from build123d import *

# Parameters (mm, degrees)
SKETCH1_R           = 25
BOSS_EXTRUDE1_DEPTH = 4
SKETCH2_R           = 1.713577746
CUT_EXTRUDE1_DEPTH  = 4
CUT_EXTRUDE2_DEPTH  = 2
SKETCH4_R           = 12.5
SKETCH4_R_2         = 3
BOSS_EXTRUDE2_DEPTH = 10
SKETCH5_R           = 1.6
CUT_EXTRUDE3_DEPTH  = 12.5
SKETCH6_R           = 3.1
CUT_EXTRUDE4_DEPTH  = 6
CUT_EXTRUDE5_DEPTH  = 3
FILLET1_R           = 1.5


with BuildPart() as part:
    # Sketch1 → Boss-Extrude1 (new body)
    with BuildSketch(Plane.XY):
        Circle(SKETCH1_R)
    extrude(amount=BOSS_EXTRUDE1_DEPTH)

    # Sketch2 → Cut-Extrude1 (cut)
    with BuildSketch(Plane(origin=(0, 0, 0), x_dir=(-1, 0, 0), z_dir=(0, 0, -1))):
        with Locations((0, 18.35)):
            Circle(SKETCH2_R)
        with Locations((15.891566159, 9.175)):
            Circle(SKETCH2_R)
        with Locations((15.891566159, -9.175)):
            Circle(SKETCH2_R)
        with Locations((0, -18.35)):
            Circle(SKETCH2_R)
        with Locations((-15.891566159, -9.175)):
            Circle(SKETCH2_R)
        with Locations((-15.891566159, 9.175)):
            Circle(SKETCH2_R)
    extrude(amount=-CUT_EXTRUDE1_DEPTH, mode=Mode.SUBTRACT)

    # Sketch3 → Cut-Extrude2 (cut)
    with BuildSketch(Plane(origin=(0, 0, 0), x_dir=(-1, 0, 0), z_dir=(0, 0, -1))):
        Polygon((13.870840217, 5.675), (17.912292102, 5.675), (19.933018044, 9.175), (17.912292102, 12.675), (13.870840217, 12.675), (11.850114275, 9.175), align=None)
        Polygon((4.041451884, 18.35), (2.020725942, 21.85), (-2.020725942, 21.85), (-4.041451884, 18.35), (-2.020725942, 14.85), (2.020725942, 14.85), align=None)
        Polygon((11.850114275, -9.175), (13.870840217, -12.675), (17.912292102, -12.675), (19.933018044, -9.175), (17.912292102, -5.675), (13.870840217, -5.675), align=None)
        Polygon((-2.020725942, -14.85), (-4.041451884, -18.35), (-2.020725942, -21.85), (2.020725942, -21.85), (4.041451884, -18.35), (2.020725942, -14.85), align=None)
        Polygon((-13.870840217, -5.675), (-17.912292102, -5.675), (-19.933018044, -9.175), (-17.912292102, -12.675), (-13.870840217, -12.675), (-11.850114275, -9.175), align=None)
        Polygon((-11.850114275, 9.175), (-13.870840217, 12.675), (-17.912292102, 12.675), (-19.933018044, 9.175), (-17.912292102, 5.675), (-13.870840217, 5.675), align=None)
    extrude(amount=-CUT_EXTRUDE2_DEPTH, mode=Mode.SUBTRACT)

    # Sketch4 → Boss-Extrude2 (add)
    with BuildSketch(Plane(origin=(0, 0, 0), x_dir=(-1, 0, 0), z_dir=(0, 0, -1))):
        with Locations(Location((0, 0, 0), (0, 0, 180))):
            Circle(SKETCH4_R)
        with Locations((0, 1)):
            Circle(SKETCH4_R_2, mode=Mode.SUBTRACT)
    extrude(amount=BOSS_EXTRUDE2_DEPTH)

    # Sketch5 → Cut-Extrude3 (cut)
    with BuildSketch(Plane(origin=(0, 12.5, 0), x_dir=(1, 0, 0), z_dir=(0, 1, 0))):
        with Locations(Location((0, 5, 0), (0, 0, 270))):
            Circle(SKETCH5_R)
    extrude(amount=-CUT_EXTRUDE3_DEPTH, mode=Mode.SUBTRACT)

    # Sketch6 → Cut-Extrude4 (cut)
    with BuildSketch(Plane(origin=(0, 12.5, 0), x_dir=(1, 0, 0), z_dir=(0, 1, 0))):
        with Locations(Location((0, 5, 0), (0, 0, 270))):
            Circle(SKETCH6_R)
    extrude(amount=-CUT_EXTRUDE4_DEPTH, mode=Mode.SUBTRACT)

    # Sketch7 → Cut-Extrude5 (cut)
    with BuildSketch(Plane(origin=(0, 1.5, 0), x_dir=(1, 0, 0), z_dir=(0, 1, 0))):
        Polygon((2.174315781, 7.9), (-12.5, 7.9), (-12.5, 2.1), (2.174315781, 2.1), (3.848631561, 5), align=None)
    extrude(amount=CUT_EXTRUDE5_DEPTH, mode=Mode.SUBTRACT)

    # Fillet1
    fillet1_edges = [part.edges().sort_by_distance(p)[0] for p in [
        (-12.5, 0, 0),
    ]]
    fillet(fillet1_edges, radius=FILLET1_R)


solid = part.part
Check sheet for the modelled part. Datum: model origin and axes. Units: mm. A direction names the side the tool comes from. Coordinates: 2 decimals unless noted, no trailing zeros. Write each loop counter-clockwise with the first axis right and the second up, starting at its lowest first coordinate (ties: lowest second). Pieces come first, ordered by that corner, then holes.
Item 1: Cross-section at B-B on x = 16. Record the boundary of the cut face in (y, z) (3 decimals).
Numbers:
outline: (-19.209, 0) - (-12.675, 0) - (-12.675, 2) - (-10.885, 2) - (-10.885, 4) - (-19.209, 4) - close; (-7.465, 2) - (-5.675, 2) - (-5.675, 0) - (5.675, 0) - (5.675, 2) - (7.465, 2) - (7.465, 4) - (-7.465, 4) - close; (10.885, 2) - (12.675, 2) - (12.675, 0) - (19.209, 0) - (19.209, 4) - (10.885, 4) - close
Item 2: Cross-section at C-C on y = 10. Count the separate pieces of the cut face and the enclosed holes in it, then the cut area to 3 significant figures.
Numbers:
separate pieces: 3
enclosed holes: 1
area: 264 mm2
Item 3: Scan lines: probe 1 along Y at (x, z) = (0, 2.5); probe 2 along Y at (x, z) = (0, 1); probe 3 along Z at (x, y) = (0, 10.5). Record each from-to range of solid material in increasing order.
Numbers:
probe 1: y = -25 to -20.06, -16.64 to 16.64, 20.06 to 25
probe 2: y = -25 to -21.85, -14.85 to 14.85, 21.85 to 25
probe 3: z = -10 to -8.1, -1.9 to 4
Item 4: Access from +Z, -Z, +X, -X, +Y, -Y to the whole of each face (thin tool, end or side, straight path). Record for faces 1 (the face through (-3.045, -16.624, 0.986)), 2 (the face through (-0.97, 5.51, -6.27)), 3 (the face through (-7, 3, -7.9)).
Numbers:
face 1: -Z
face 2: +Y
face 3: -X
Item 5: Mould release check, pull along Y, two halves, no side actions. Record for faces 4 (the face through (0, -14.85, 1)), 5 (the face through (3.074, 9.542, -5.404)): released by +Y, released by -Y, zero draft, split by the parting line, or undercut.
Numbers:
face 4: undercut
face 5: zero draft
Item 6: Depth check by flat-ended pin: pin 1 Ø2.5 at (x, z) = (0, -5) entering from +Y; pin 2 Ø1.6 at (x, z) = (15.5, 1.5) entering from -Y; pin 3 Ø4 at (x, y) = (0, 18.35) entering from -Z. Enter the tip coordinate at first touch or a pass-through.
Numbers:
pin 1: stops at y = -1.73
pin 2: stops at y = -20.22
pin 3: stops at z = 2
Item 7: Cross-section at A-A on z = 3. Record the boundary of the cut face in (x, y) (3 decimals).
Numbers:
outline: circle Ø50 at (0, 0); hole circle Ø3.427 at (-15.892, -9.175); hole circle Ø3.427 at (-15.892, 9.175); hole circle Ø3.427 at (0, -18.35); hole circle Ø3.427 at (0, 18.35); hole circle Ø3.427 at (15.892, -9.175); hole circle Ø3.427 at (15.892, 9.175)
